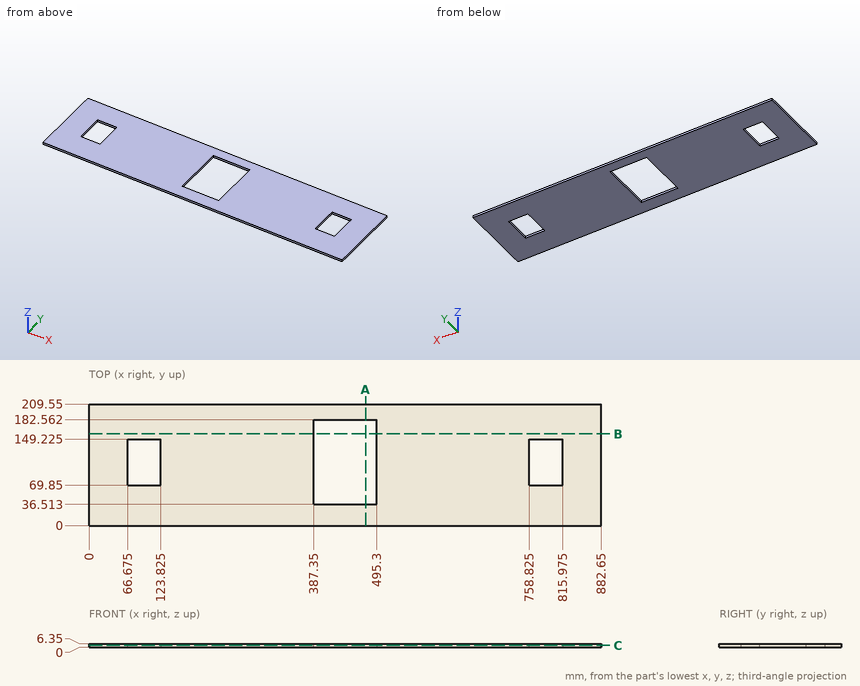
The drawing under review shows one solid part. Ordinate dimensions are in mm from its lowest x, y, z. Coordinates: 2 decimals unless noted, no trailing zeros. Order: outer loops, then holes, each group sorted by start corner. A loop starts at its lowest first (then second) coordinate and runs counter-clockwise, first axis right, second up. Notation, with made-up numbers: (25, 16) -> (62, 16) arc R25 cw to (62, 50) -> close; hole circle Ø5 at (75, -31.5). An arc over 180 degrees is marked (long way). Answer in a Markdown table with one row per item.
(1) Wall thickness on line 1 along X through (y, z) = (37.5, 3.25); line 2 along Y through (x, z) = (484.5, 5.5): over which ranges is each line inside the solid? List them lowest first.
Answers:
| item | result |
|---|---|
| line 1 | 0 to 387.35, 495.3 to 882.65 |
| line 2 | 0 to 36.51, 182.56 to 209.55 |
(2) Consider section A-A (x = 476.5). Write out the cut boundary in (y, z), plus the area to 3 significant figures.
Answers:
| item | result |
|---|---|
| outline | (0, 0) -> (36.51, 0) -> (36.51, 6.35) -> (0, 6.35) -> close; (182.56, 0) -> (209.55, 0) -> (209.55, 6.35) -> (182.56, 6.35) -> close |
| area | 403 mm² |
(3) Consider section C-C (z = 3.5). State how many separate pieces and enclosed holes the cut face has, plus the area to 3 significant figures.
Answers:
| item | result |
|---|---|
| separate pieces | 1 |
| enclosed holes | 3 |
| area | 160,000 mm² |
(4) Consider section B-B (y = 158). Write out the cut boundary in (x, z), plus the area to 3 significant figures.
Answers:
| item | result |
|---|---|
| outline | (0, 0) -> (387.35, 0) -> (387.35, 6.35) -> (0, 6.35) -> close; (495.3, 0) -> (882.65, 0) -> (882.65, 6.35) -> (495.3, 6.35) -> close |
| area | 4,920 mm² |
